Check sheet for the modelled part. Datum: model origin and axes. Units: mm. A direction names the side the tool comes from. Give positions to 0.01 mm unless a question says otherwise; leave off trailing zeros. Order: outer loops, then holes, each group sorted by start corner. A loop starts at its lowest first (then second) coordinate and runs counter-clockwise, first axis right, second up. Notation, with made-up numbers: M -15,53 L 18,53 A24 cw 18,71 Z; hole C 68.25,59.25 d9. An arc over 180 degrees is marked long. Return JSON: item names as keys, results as strings. Group by question number.
Autodesk Fusion 360 part; units mm, degrees
sketch "Sketch1" plane through (0, 0, 0) normal (0, 1, 0) x (1, 0, 0) in component "BNC 4-hole panel mount"
  line L0 (-6.35, -9.3) -> (-8.75, -9.3)
  line L1 (-8.75, -9.3) -> (-8.75, -11.6)
  line L2 (-8.75, -11.6) -> (-6.35, -11.6)
  line L3 (-6.35, -11.6) -> (-6.35, -16.6)
  line L4 (-6.35, -16.6) -> (-4.85, -16.6)
  line L5 (-4.85, -16.6) -> (-4.85, -27.6)
  line L6 (0, -27.6) -> (0, 0)
  line L7 (-6.35, -9.3) -> (-6.35, -7.3)
  line L8 (-6.35, -7.3) -> (-1.9, -7.3)
  line L9 (-1.9, -7.3) -> (-1.9, 0)
  line L10 (0, 0) -> (-1.9, 0)
  line L11 (-4.85, -27.6) -> (-4.35, -27.6)
  line L12 (-4.35, -27.6) -> (-4.35, -14.6)
  line L13 (-4.35, -14.6) -> (-0.6, -14.6)
  line L14 (-0.6, -14.6) -> (-0.6, -24.1)
  line L15 (-0.6, -24.1) -> (0, -25.6)
  dimension "d3" = 1.9
  dimension "d4" = 2.3
  dimension "d5" = 5
  dimension "d6" = 8.75
  dimension "d9" = 4.85
  dimension "d10" = 6.35
  dimension "d11" = 2
  dimension "d21" = 0.5
  dimension "d22" = 0.6
  dimension "d23" = 1.5
  dimension "d24" = 13
  dimension "d25" = 27.6
  dimension "d26" = 11
  dimension "d27" = 16
revolve "Revolve1" add sketch "Sketch1" angle 360 about axis through (0, 0, 27.6) along (0, 0, -1) in component "BNC 4-hole panel mount"
sketch "Sketch2" plane through (0, 0, 11.6) normal (0, 0, 1) x (-1, 0, 0) in component "BNC 4-hole panel mount"
  circle A0 centre (0, 0) radius 6.35
  circle A1 centre (0, 0) radius 8.75
  line L0 (8.75, -8.75) -> (-8.75, -8.75)
  line L1 (-8.75, -8.75) -> (-8.75, 8.75)
  line L2 (-8.75, 8.75) -> (8.75, 8.75)
  line L3 (8.75, 8.75) -> (8.75, -8.75)
  line L4 (8.75, -8.75) -> (-8.75, 8.75) construction
  line L5 (-8.75, -8.75) -> (8.75, 8.75) construction
  circle A2 centre (6.35, 6.35) radius 1.6
  circle A3 centre (6.35, -6.35) radius 1.6
  circle A4 centre (-6.35, -6.35) radius 1.6
  circle A5 centre (-6.35, 6.35) radius 1.6
  circle A6 centre (0, 0) radius 6.35
  dimension "d13" = 17.5
  dimension "d14" = 17.5
  dimension "d15" = 3.2
  dimension "d16" = 12.7
extrude "Extrude1" add sketch "Sketch2" against normal up to surface (2.3 mm away) contours A1 A2 A3 A4 A5 | A1 L0 L3 A3 | A1 L2 L3 A2 | A1 L1 L2 A5 | A1 L0 L1 A4 in component "BNC 4-hole panel mount"
extrude "Extrude2" cut sketch "Sketch2" against normal up to surface (2.3 mm away) contours A1 A2 | A1 A3 | A1 A5 | A1 A4 picked at (5.857, 5.857) picked at (6.6353, -6.5855) picked at (-6.6375, 6.5831) picked at (-5.8818, -5.8337) in component "BNC 4-hole panel mount"
chamfer "Chamfer1" distance 1.5 angle 45 4 edges at (8.75, -8.75, 10.45) (-8.75, -8.75, 10.45) (-8.75, 8.75, 10.45) (8.75, 8.75, 10.45) in component "BNC 4-hole panel mount"
component "BNC 4-hole panel mount" placed x (1, 0, 0) y (0, 1, 0) z (0, 0, 1) at (0, 0, 0)
equation "d14 = d13"
1) Sectioned sample at C-C on x = 4. Record the boundary of the cut face in (y, z), then the cut area to 3 significant figures.
2) Depth check by flat-ended pin: P1, Ø4, axis at y = -5, z = 16.5, coming from the -X side; P2, Ø3, axis at x = 6.35, y = 6.35, coming from the +Z side; P3, Ø6.5, axis at x = -1.5, y = 1.5, coming from the -Z side; P4, Ø4, axis at x = -6.35, y = -6.35, coming from the +Z side. Enter the tip coordinate at first touch or a pass-through.
3) Sectioned sample at B-B on x = -5.75. Record the boundary of the cut face in (y, z), then the cut area to 3 significant figures.
4) Tool access check on faces 1 (the face through (6.172, -6.203, 10.466)), 2 (the face through (0.943, -4.247, 21.009)), 3 (the face through (-1, 2, 7.3)). Record the directions out of +Z, -Z, +X, -X, +Y, -Y that give a thin tool (end or side, any length) a straight path to the whole face; none if there is none.
5) Sectioned sample at A-A on z = 21. Record the boundary of the cut face in (x, y).
6) Material ranges on line 1 along X through (y, z) = (6.35, 10.25); line 2 along X through (y, z) = (-6.35, 10.6), recorded low to high.
7) Sectioned sample at D-D on z = 13. Record the boundary of the cut face in (x, y).
Reply:
{
 "1": {"outline": "M -8.75,9.3 L -4.93,9.3 L -4.93,7.3 L 4.93,7.3 L 4.93,9.3 L 8.75,9.3 L 8.75,11.6 L 4.93,11.6 L 4.93,16.6 L 2.74,16.6 L 2.74,27.6 L 1.71,27.6 L 1.71,14.6 L -1.71,14.6 L -1.71,27.6 L -2.74,27.6 L -2.74,16.6 L -4.93,16.6 L -4.93,11.6 L -8.75,11.6 Z", "area": "125 mm^2"},
 "2": {"P1": "x = -5.6", "P2": "through", "P3": "z = 0", "P4": "z = 11.6"},
 "3": {"outline": "M -8.75,9.3 L -7.83,9.3 L -7.83,11.6 L -8.75,11.6 Z; M -4.87,9.3 L -2.69,9.3 L -2.69,7.3 L 2.69,7.3 L 2.69,9.3 L 6.6,9.3 L 6.6,11.6 L 2.69,11.6 L 2.69,16.6 L -2.69,16.6 L -2.69,11.6 L -4.87,11.6 Z; M 7.83,9.3 L 8.75,9.3 L 8.75,11.6 L 7.83,11.6 Z", "area": "68.3 mm^2"},
 "4": {"face 1": "+Z, -Z", "face 2": "+Z", "face 3": "-Z"},
 "5": {"outline": "C 0,0 d9.7; C 0,0 d1.2; hole C 0,0 d8.7"},
 "6": {"line 1": "-8.75 to -7.95, -6.02 to 4.75, 7.95 to 8.75", "line 2": "-8.75 to -7.95, -4.75 to 6.02, 7.95 to 8.75"},
 "7": {"outline": "C 0,0 d12.7"}
}
